Autodesk Fusion 360 part; units mm, degrees
sketch "Sketch1" plane through (0, 0, 0) normal (0, 0, 1) x (1, 0, 0)
  line L0 (-33.85, 45.35) -> (33.85, 45.35)
  line L1 (33.85, 45.35) -> (33.85, -45.35)
  line L2 (33.85, -45.35) -> (-33.85, -45.35)
  line L3 (-33.85, -45.35) -> (-33.85, 45.35)
  line L4 (0, 0) -> (-33.85, 0)
  line L5 (0, 0) -> (0, 45.35)
  dimension "d13" = 90.7
  dimension "d14" = 67.7
extrude "Extrude1" add sketch "Sketch1" along normal blind 4
sketch "Sketch3" plane through (0, 0, 4) normal (0, 0, 1) x (-1, 0, 0)
  line L0 (1.875, -19.5) -> (-1.875, -19.5)
  line L1 (-1.875, -19.5) -> (-1.875, -0.6092)
  line L2 (-1.875, -0.6092) -> (-12.9787, 14.6737)
  line L3 (-12.9787, 14.6737) -> (-9.9449, 16.8779)
  line L4 (-9.9449, 16.8779) -> (0, 3.1899)
  line L5 (0, 3.1899) -> (9.9449, 16.8779)
  line L6 (9.9449, 16.8779) -> (12.9787, 14.6737)
  line L7 (12.9787, 14.6737) -> (1.875, -0.6092)
  line L8 (1.875, -0.6092) -> (1.875, -19.5)
  line L9 (0, -19.5) -> (0, 0)
  line L10 (0, 0) -> (-11.4618, 15.7758)
  line L11 (11.4618, 15.7758) -> (0, 0)
  line L12 (33.85, 45.35) -> (-33.85, 45.35)
  line L13 (-33.85, 45.35) -> (-33.85, -45.35)
  line L14 (-33.85, -45.35) -> (33.85, -45.35)
  line L15 (33.85, -45.35) -> (33.85, 45.35)
  dimension "d7" = 144
  dimension "d8" = 144
  dimension "d9" = 3.75
  dimension "d10" = 19.5
extrude "Extrude3" add sketch "Sketch3" along normal blind 50 contours L0 L6 L7 L8 L9 L11 | L0 L1 L2 L3 L9 L10 | L3 L4 L5 L6 L10 L11
Source: CAD feature listing. Evaluate the final solid. Frame: model axes, mm. A direction names the side the tool comes from. Give positions to 0.01 mm unless a question says otherwise; leave off trailing zeros. Order: outer loops, then holes, each group sorted by start corner. A loop starts at its lowest first (then second) coordinate and runs counter-clockwise, first axis right, second up. Notation, with made-up numbers: (46, 76) -> (100, 76) arc R38 ccw to (100, 114) -> close; hole circle Ø11 at (31.5, -30). An arc over 180 degrees is marked (long way). Use a Markdown table: item, result.
Q1. Section C-C (x = 17). Return the cut outline in (y, z).
A:
| item | result |
|---|---|
| outline | (-45.35, 0) -> (45.35, 0) -> (45.35, 4) -> (-45.35, 4) -> close |
Q2. Material intervals for line 1 (Z direction, x = -5, y = 35); line 2 (X direction, y = -9.5, z = 5.5); line 3 (X direction, y = 6, z = 8.5) (3 decimals), sorted ascending. Write a range as [from, to].
A:
| item | result |
|---|---|
| line 1 | [0, 4] |
| line 2 | [-9.22, -4.58], [4.58, 9.22] |
| line 3 | [-1.875, 1.875] |
Q3. Pull-direction query (X, two-part tool) for faces 1 (the face through (5.04, -10.13, 28.65)), 2 (the face through (-11.44, -15.79, 28.65)), 3 (the face through (0, -1, 54)), 4 (the face through (7.349, -6.925, 28.65)); classes: +X half, -X half, draft (parallel to the pull), parting line (faces both ways), or undercut.
A:
| item | result |
|---|---|
| face 1 | undercut |
| face 2 | -X half |
| face 3 | draft |
| face 4 | +X half |
Q4. Section B-B (y = 24.5). Return the cut outline in (x, z), and give its area (3 significant figures).
A:
| item | result |
|---|---|
| outline | (-33.85, 0) -> (33.85, 0) -> (33.85, 4) -> (-33.85, 4) -> close |
| area | 271 mm^2 |
Q5. Section D-D (y = -12.5). Return the cut outline in (x, z), and give its area (3 significant figures).
A:
| item | result |
|---|---|
| outline | (-33.85, 0) -> (33.85, 0) -> (33.85, 4) -> (11.4, 4) -> (11.4, 54) -> (6.76, 54) -> (6.76, 4) -> (-6.76, 4) -> (-6.76, 54) -> (-11.4, 54) -> (-11.4, 4) -> (-33.85, 4) -> close |
| area | 734 mm^2 |
Q6. First-contact query: P1, Ø3, axis at x = 0, z = 29.5, coming from the +Y side; P2, Ø3, axis at x = 1, z = 44, coming from the -Y side; P3, Ø1, axis at x = 25, y = 36, coming from the -Z side; P4, Ø1, axis at x = 7.5, z = 40, coming from the +Y side. Flat tips, straight axial feed; report the tip coordinate or a pass-through.
A:
| item | result |
|---|---|
| P1 | y = 19.5 |
| P2 | y = -6.63 |
| P3 | z = 0 |
| P4 | y = -6.44 |
Q7. Section A-A (z = 9). Return the cut outline in (x, y) (3 decimals).
A:
| item | result |
|---|---|
| outline | (-12.979, -14.674) -> (-9.945, -16.878) -> (0, -3.19) -> (9.945, -16.878) -> (12.979, -14.674) -> (1.875, 0.609) -> (1.875, 19.5) -> (-1.875, 19.5) -> (-1.875, 0.609) -> close |
Q8. Access query for faces 5 (the face through (0, 19.5, 29)), 6 (the face through (1.875, 10, 29)), 7 (the face through (-7.505, -7.139, 28.65)), 8 (the face through (11.483, -15.76, 28.65)). Directions: +Z, -Z, +X, -X, +Y, -Y. A direction counts if a zero-diameter tool reaches every point of the face in a straight line with its end or side. Return the directions, or none.
A:
| item | result |
|---|---|
| face 5 | +Z, +X, -X, +Y |
| face 6 | +Z, +X, +Y |
| face 7 | +Z, -X, +Y |
| face 8 | +Z, +X, -Y |
